from build123d import *

# Parameters (mm, degrees)
SKETCH1_R           = 250
SKETCH1_R_2         = 39
BOSS_EXTRUDE1_DEPTH = 3
SKETCH2_R           = 40
SKETCH2_R_2         = 39
BOSS_EXTRUDE2_DEPTH = 100
SKETCH3_R           = 77.5
SKETCH3_R_2         = 72.5
BOSS_EXTRUDE3_DEPTH = 100


with BuildPart() as part:
    # Sketch1 → Boss-Extrude1 (new body)
    with BuildSketch(Plane(origin=(0, 0, 0), x_dir=(1, 0, 0), z_dir=(0, 1, 0))):
        with Locations(Location((0, 0, 0), (0, 0, 270))):
            Circle(SKETCH1_R)
        with Locations(Location((141.421356237, 141.421356237, 0), (0, 0, 270))):
            Circle(SKETCH1_R_2, mode=Mode.SUBTRACT)
        with Locations(Location((-141.421356237, 141.421356237, 0), (0, 0, 90))):
            Circle(SKETCH1_R_2, mode=Mode.SUBTRACT)
        with Locations(Location((-141.421356237, -141.421356237, 0), (0, 0, 270))):
            Circle(SKETCH1_R_2, mode=Mode.SUBTRACT)
        with Locations(Location((141.421356237, -141.421356237, 0), (0, 0, 90))):
            Circle(SKETCH1_R_2, mode=Mode.SUBTRACT)
        with Locations(Location((0, 200, 0), (0, 0, 270))):
            Circle(SKETCH1_R_2, mode=Mode.SUBTRACT)
        with Locations(Location((200, 0, 0), (0, 0, 90))):
            Circle(SKETCH1_R_2, mode=Mode.SUBTRACT)
        with Locations(Location((0, -200, 0), (0, 0, 270))):
            Circle(SKETCH1_R_2, mode=Mode.SUBTRACT)
        with Locations(Location((-200, 0, 0), (0, 0, 270))):
            Circle(SKETCH1_R_2, mode=Mode.SUBTRACT)
    extrude(amount=BOSS_EXTRUDE1_DEPTH)

    # Sketch2 → Boss-Extrude2 (add)
    # profile 1 of 8: a face of its own
    with BuildSketch(Plane(origin=(0, 3, 0), x_dir=(1, 0, 0), z_dir=(0, 1, 0))):
        with Locations(Location((0, 200, 0), (0, 0, 270))):
            Circle(SKETCH2_R)
        with Locations(Location((0, 200, 0), (0, 0, 270))):
            Circle(SKETCH2_R_2, mode=Mode.SUBTRACT)
    # profile 2 of 8: a face of its own
    with BuildSketch(Plane(origin=(0, 3, 0), x_dir=(1, 0, 0), z_dir=(0, 1, 0))):
        with Locations(Location((141.421356237, 141.421356237, 0), (0, 0, 270))):
            Circle(SKETCH2_R)
        with Locations(Location((141.421356237, 141.421356237, 0), (0, 0, 270))):
            Circle(SKETCH2_R_2, mode=Mode.SUBTRACT)
    # profile 3 of 8: a face of its own
    with BuildSketch(Plane(origin=(0, 3, 0), x_dir=(1, 0, 0), z_dir=(0, 1, 0))):
        with Locations(Location((200, 0, 0), (0, 0, 270))):
            Circle(SKETCH2_R)
        with Locations(Location((200, 0, 0), (0, 0, 90))):
            Circle(SKETCH2_R_2, mode=Mode.SUBTRACT)
    # profile 4 of 8: a face of its own
    with BuildSketch(Plane(origin=(0, 3, 0), x_dir=(1, 0, 0), z_dir=(0, 1, 0))):
        with Locations(Location((141.421356237, -141.421356237, 0), (0, 0, 270))):
            Circle(SKETCH2_R)
        with Locations(Location((141.421356237, -141.421356237, 0), (0, 0, 90))):
            Circle(SKETCH2_R_2, mode=Mode.SUBTRACT)
    # profile 5 of 8: a face of its own
    with BuildSketch(Plane(origin=(0, 3, 0), x_dir=(1, 0, 0), z_dir=(0, 1, 0))):
        with Locations(Location((0, -200, 0), (0, 0, 270))):
            Circle(SKETCH2_R)
        with Locations(Location((0, -200, 0), (0, 0, 270))):
            Circle(SKETCH2_R_2, mode=Mode.SUBTRACT)
    # profile 6 of 8: a face of its own
    with BuildSketch(Plane(origin=(0, 3, 0), x_dir=(1, 0, 0), z_dir=(0, 1, 0))):
        with Locations(Location((-141.421356237, -141.421356237, 0), (0, 0, 270))):
            Circle(SKETCH2_R)
        with Locations(Location((-141.421356237, -141.421356237, 0), (0, 0, 270))):
            Circle(SKETCH2_R_2, mode=Mode.SUBTRACT)
    # profile 7 of 8: a face of its own
    with BuildSketch(Plane(origin=(0, 3, 0), x_dir=(1, 0, 0), z_dir=(0, 1, 0))):
        with Locations(Location((-200, 0, 0), (0, 0, 270))):
            Circle(SKETCH2_R)
        with Locations(Location((-200, 0, 0), (0, 0, 270))):
            Circle(SKETCH2_R_2, mode=Mode.SUBTRACT)
    # profile 8 of 8: a face of its own
    with BuildSketch(Plane(origin=(0, 3, 0), x_dir=(1, 0, 0), z_dir=(0, 1, 0))):
        with Locations(Location((-141.421356237, 141.421356237, 0), (0, 0, 270))):
            Circle(SKETCH2_R)
        with Locations(Location((-141.421356237, 141.421356237, 0), (0, 0, 90))):
            Circle(SKETCH2_R_2, mode=Mode.SUBTRACT)
    extrude(amount=BOSS_EXTRUDE2_DEPTH)

    # Sketch3 → Boss-Extrude3 (add)
    with BuildSketch(Plane(origin=(0, 3, 0), x_dir=(1, 0, 0), z_dir=(0, 1, 0))):
        with Locations(Location((0, 0, 0), (0, 0, 270))):
            Circle(SKETCH3_R)
        with Locations(Location((0, 0, 0), (0, 0, 270))):
            Circle(SKETCH3_R_2, mode=Mode.SUBTRACT)
    extrude(amount=BOSS_EXTRUDE3_DEPTH)


solid = part.part
Verification items for the finished model (mm, model axes). A direction names the side the tool comes from. Coordinates: 2 decimals unless noted, no trailing zeros. Loops run counter-clockwise (first coordinate to the right, second up) from the corner with the lowest first, then second, coordinate; pieces in that order, holes last. Notation, with made-up numbers: (32.5, 54) -> (46.5, 54) arc R14 cw to (46.5, 64) -> close; hole circle Ø11 at (51.25, 68.5). An arc over 180 degrees is marked (long way). Answer as a JSON object with one key per item and string values. Group by question number.
Item 1: Depth check by flat-ended pin: pin 1 (10 mm diameter, centred on y = 47.5, z = -131, fed in from -X); pin 2 (4 mm diameter, centred on x = 35, y = 76, fed in from +Z); pin 3 (1.5 mm diameter, centred on y = 56, z = 33, fed in from -X). Enter the tip coordinate at first touch or a pass-through.
Item 2: Sectioned sample at C-C on y = 41. State how many separate pieces and enclosed holes the cut face has, plus the area to 3 significant figures.
Item 3: Sectioned sample at D-D on z = 0. Record the boundary of the cut face in (x, y), plus the area to 3 significant figures.
Item 4: Sectioned sample at B-B on x = 200. Record the boundary of the cut face in (y, z), plus the area to 3 significant figures.
Item 5: Scan lines: probe 1 along Z at (x, y) = (201, 93.5); probe 2 along Z at (x, y) = (123.5, 51); probe 3 along Z at (x, y) = (114, 16). Record each from-to range of solid material in increasing order.
Item 6: Mould release check, pull along Z, two halves, no side actions. Record for faces 1 (the flat face through (1, 3, -1)), 2 (the flat face through (191.3, 103, 38.3)): +Z half, -Z half, draft (parallel to the pull), parting line (faces both ways), or undercut.
Item 7: Tool access check on faces 3 (the cylindrical face through (160.95, 52.3, -8.67)), 4 (the flat face through (-38.3, 103, 208.7)). Record the directions out of +Z, -Z, +X, -X, +Y, -Y that give a thin tool (end or side, any length) a straight path to the whole face; none if there is none.
Item 8: Sectioned sample at A-A on z = -200. Record the boundary of the cut face in (x, y), plus the area to 3 significant figures.
Evaluation:
{
 "1": {"pin 1": "stops at x = -181.05", "pin 2": "stops at z = 222.61", "pin 3": "stops at x = -223.66"},
 "2": {"separate pieces": "9", "enclosed holes": "9", "area": "4,340 mm²"},
 "3": {"outline": "(-250, 0) -> (-239, 0) -> (-239, 103) -> (-240, 103) -> (-240, 3) -> (-250, 3) -> close; (-161, 0) -> (161, 0) -> (161, 103) -> (160, 103) -> (160, 3) -> (77.5, 3) -> (77.5, 103) -> (72.5, 103) -> (72.5, 3) -> (-72.5, 3) -> (-72.5, 103) -> (-77.5, 103) -> (-77.5, 3) -> (-160, 3) -> (-160, 103) -> (-161, 103) -> close; (239, 0) -> (250, 0) -> (250, 3) -> (240, 3) -> (240, 103) -> (239, 103) -> close", "area": "2,430 mm²"},
 "4": {"outline": "(0, -150) -> (3, -150) -> (3, -40) -> (103, -40) -> (103, -39) -> (0, -39) -> close; (0, 39) -> (103, 39) -> (103, 40) -> (3, 40) -> (3, 150) -> (0, 150) -> close", "area": "866 mm²"},
 "5": {"probe 1": "z = -39.99 to -38.99, 38.99 to 39.99", "probe 2": "z = -177.18 to -176.06, -106.78 to -105.66, 105.66 to 106.78, 176.06 to 177.18", "probe 3": "z = -170.54 to -169.15, -113.69 to -112.3, 112.3 to 113.69, 169.15 to 170.54"},
 "6": {"face 1": "undercut", "face 2": "draft"},
 "7": {"face 3": "+Y", "face 4": "+Z, -Z, +X, -X, +Y"},
 "8": {"outline": "(-150, 0) -> (-39, 0) -> (-39, 103) -> (-40, 103) -> (-40, 3) -> (-150, 3) -> close; (39, 0) -> (150, 0) -> (150, 3) -> (40, 3) -> (40, 103) -> (39, 103) -> close", "area": "866 mm²"}
}
